Verification items for the finished model (mm, model axes). A direction names the side the tool comes from. Coordinates: 2 decimals unless noted, no trailing zeros. Order: outer loops, then holes, each group sorted by start corner. A loop starts at its lowest first (then second) coordinate and runs counter-clockwise, first axis right, second up. Notation, with made-up numbers: (23, -38) -> (79, -38) arc R17 cw to (79, -6) -> close; hole circle Ø7 at (54.5, 7.5). An arc over 180 degrees is marked (long way). Write item = value, one per line. Start each with the question number.
1. Cross-section at C-C on x = 0.5. Record the cut outline in (y, z).
2. Set-up check for faces 4 (the flat face through (0, -1.7, -3.2)), 5 (the flat face through (2, -3, -2)): record each of +Z, -Z, +X, -X, +Y, -Y from which the full face is reachable in a straight line by a thin tool's end or side.
3. Go/stop test with flat-tipped pins: P1, Ø3, axis at y = -2.5, z = -1.5, coming from the +X side; P2, Ø3, axis at x = 23, z = 2, coming from the -Y side; P3, Ø1, axis at x = 22.5, z = -5, coming from the +Y side; P4, Ø1, axis at x = -1, z = -4.5, coming from the +Y side. Record where each tip stops, or that it passes through.
4. Release check for a two-part mould opening along X. For faces 1 (the flat face through (30, -5, -5)), 2 (the cylindrical face through (7.948, -6.016, 5.73)), 3 (the cylindrical face through (-3.04, -0.15, 0.98)) record: +X half, -X half, draft (parallel to the pull), parting line (faces both ways), or undercut.
5. Cross-section at B-B on z = -1. Record the cut outline in (x, y).
6. Cross-section at A-A on y = -3.25. Give the number of separate pieces and of enclosed holes in the cut face, plus the area to 3 significant figures.
7. Cross-section at D-D on x = 14. Record the cut outline in (y, z).
8. Thickness scan on line 1 along Z through (x, y) = (20, -3.25); line 2 along X through (y, z) = (-4.75, 5); line 3 along Z through (x, y) = (-3.25, -3.25). Record the ranges inside material, lowest first. Write a range as from..to.
from build123d import *

# Parameters (mm, degrees)
F_6_0_6_DIAMETER_HOLE3_D           = 6
F_6_0_6_DIAMETER_HOLE3_ON_FACE_2_D = 6
SKETCH7_R                          = 5
CUT_EXTRUDE1_DEPTH                 = 28


with BuildPart() as part:
    # Sketch1 → Revolve2 (revolve)
    with BuildSketch(Plane.XY):
        Polygon((0, 0), (-6, 0), (-6, -1.5), (2, -1.5), (2, 0.25), (28, 0.25), (28, -3.25), (30, -3.25), (30, 4.25), (0, 4.25), align=None)
    revolve(axis=Axis((-6, -3.25, 0), (1, 0, 0)))

    # Ø6.0 (6) Diameter Hole3 (through all)
    with Locations(Plane(origin=(6.798989942, -3.243014935, 7.499996747), x_dir=(0, 0.999999566, -0.000931342), z_dir=(0, 0.000931342, 0.999999566))):
        with Locations((0, 0)):
            Hole(F_6_0_6_DIAMETER_HOLE3_D / 2)

    # Ø6.0 (6) Diameter Hole3 on face 2 (through all)
    with Locations(Plane(origin=(14.798989942, -3.243014935, 7.499996747), x_dir=(0, 0.999999567, -0.000931), z_dir=(0, 0.000931, 0.999999567))):
        with Locations((0, 0)):
            Hole(F_6_0_6_DIAMETER_HOLE3_ON_FACE_2_D / 2)

    # Sketch7 → Cut-Extrude1 (cut)
    with BuildSketch(Plane(origin=(30, 0, 0), x_dir=(0, 0, -1), z_dir=(1, 0, 0))):
        with Locations((0, -3.25)):
            Circle(SKETCH7_R)
    extrude(amount=-CUT_EXTRUDE1_DEPTH, mode=Mode.SUBTRACT)


solid = part.part
Worked out:
q1.outline = circle Ø15 at (-3.25, 0); hole circle Ø3.5 at (-3.25, 0)
q2.face_4 = -X
q2.face_5 = +X
q3.P1 = 2
q3.P2 = -10.73
q3.P3 = 2.75
q3.P4 = through
q4.face_1 = +X half
q4.face_2 = undercut
q4.face_3 = draft
q5.outline = (-6, -6.34) -> (0, -6.34) -> (0, -10.68) -> (30, -10.68) -> (30, -8.15) -> (2, -8.15) -> (2, -4.69) -> (-6, -4.69) -> close; (-6, -1.81) -> (2, -1.81) -> (2, 1.65) -> (30, 1.65) -> (30, 4.18) -> (0, 4.18) -> (0, -0.16) -> (-6, -0.16) -> close
q6.separate_pieces = 6
q6.enclosed_holes = 0
q6.area = 121 mm²
q7.outline = (-6.15, -6.92) -> (-6.15, -4.08) arc R5 cw to (-6.14, 4.08) -> (-6.14, 6.92) arc R7.5 ccw to start; (-0.36, -6.92) arc R7.5 ccw to (-0.35, 6.92) -> (-0.35, 4.08) arc R5 cw to (-0.36, -4.08) -> close
q8.line_1 = -7.5..-5, 5..7.5
q8.line_2 = 0..4.2, 9.39..12.2, 17.39..30
q8.line_3 = -3.25..-1.75, 1.75..3.25
